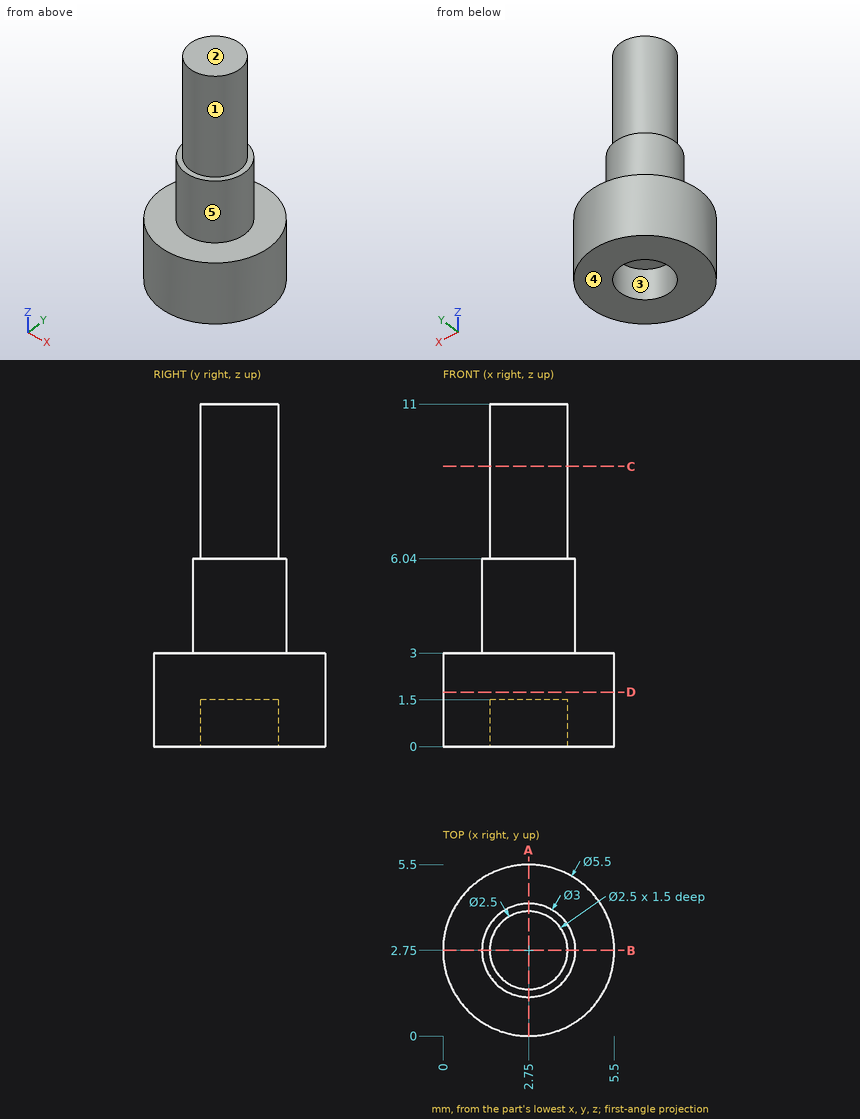
Geometry check sheet. Reference: drawing and pictorial views, mm from the part's lowest x, y, z. A direction names the side the tool comes from. Coordinates: 2 decimals unless noted, no trailing zeros. Order: outer loops, then holes, each group sorted by start corner. A loop starts at its lowest first (then second) coordinate and runs counter-clockwise, first axis right, second up. Notation, with made-up numbers: (-19.75, -16) - (-15.75, -16) arc R21 cw to (-15.75, 23) - close; hole circle Ø9 at (72.25, -4.5). An arc over 180 degrees is marked (long way). Answer in a Markdown table with one row per item. Add a question column.
1) Gauge pin test, flat ends, axial feed: P1, Ø1.5, axis at x = 4.5, z = 9, coming from the -Y side; P2, Ø1.5, axis at y = 2, z = 2, coming from the +X side; P3, Ø1, axis at y = 3, z = 8.5, coming from the +X side; P4, Ø2, axis at y = 1.5, z = 3.5, coming from the -X side. Record the tip position at first contact, or that the pin passes through.
2) Material ranges on line 1 along Y through (x, z) = (2.75, 0.8); line 2 along Z through (x, y) = (3.7, 1.3); line 3 along Z through (x, y) = (3.35, 4), recorded low to high. Write a range as [from, to].
3) Cross-section at C-C, the plane z = 9. Record the cut outline in (x, y).
4) Release check for a two-part mould opening along X. For the marked faces 3, 4 and 5 record: +X half, -X half, draft (parallel to the pull), parting line (faces both ways), or undercut.
5) Cross-section at A-A, the plane x = 2.75. Record the cut outline in (y, z).
6) Cross-section at D-D, the plane z = 1.75. Record the cut outline in (x, y), then the cut area to 3 significant figures.
7) Set-up check for the marked faces 1 and 2: record each of +Z, -Z, +X, -X, +Y, -Y from which the full face is reachable in a straight line by a thin tool's end or side.
Check result:
| question | item | result |
|---|---|---|
| 1 | P1 | stops at y = 2 |
| 1 | P2 | stops at x = 5.5 |
| 1 | P3 | stops at x = 4 |
| 1 | P4 | stops at x = 0.03 |
| 2 | line 1 | y = [0, 1.5], [4, 5.5] |
| 2 | line 2 | z = [0, 3] |
| 2 | line 3 | z = [0, 6.04] |
| 3 | outline | circle Ø2.5 at (2.75, 2.75) |
| 4 | face 3 | undercut |
| 4 | face 4 | draft |
| 4 | face 5 | parting line |
| 5 | outline | (0, 0) - (1.5, 0) - (1.5, 1.5) - (4, 1.5) - (4, 0) - (5.5, 0) - (5.5, 3) - (4.25, 3) - (4.25, 6.04) - (4, 6.04) - (4, 11) - (1.5, 11) - (1.5, 6.04) - (1.25, 6.04) - (1.25, 3) - (0, 3) - close |
| 6 | outline | circle Ø5.5 at (2.75, 2.75) |
| 6 | area | 23.8 mm² |
| 7 | face 1 | +Z |
| 7 | face 2 | +Z, +X, -X, +Y, -Y |
